Build history of the part. All positions in model axes, mm. Coordinates: 2 decimals unless noted, no trailing zeros. Loops run counter-clockwise (first coordinate to the right, second up) from the corner with the lowest first, then second, coordinate; pieces in that order, holes last.
Item 1: Cut at C-C (z = -2.5). List the corners of the cut face in (x, y), and give its area (3 significant figures).
Item 2: Cut at D-D (x = -1.5). List the corners of the cut face in (y, z), and give its area (3 significant figures).
Item 3: Flat gauge pin, fed straight in: pin 1 (2.5 mm diameter, centred on y = 0, z = 0, fed in from -X). Where does the tip first touch, or does it go through?
Item 4: Cut at A-A (y = -1). List the corners of the cut face in (x, z).
Item 5: Cut at B-B (z = 0.2). List the corners of the cut face in (x, y), and give its area (3 significant figures).
Item 6: Drill centre lines: line 1 along Z through (x, y) = (-1.1, -0.75); line 2 along Y through (x, z) = (1, 0); line 3 along Y through (x, z) = (-0.4, 0). Where is each one in solid material? Low to high.
from build123d import *
from build123d.topology import SkipClean

# Parameters (mm, degrees)
CUT_EXTRUDE_1_DEPTH      = 10
CUT_EXTRUDE_1_DEPTH_BACK = 10
SKETCH_2_W               = 8.130865192
SKETCH_2_H               = 8.836363256
SKETCH_2_W_2             = 5
SKETCH_2_H_2             = 6.113384394
SKETCH_3_R               = 1.5
CUT_EXTRUDE_2_DEPTH      = 10


with BuildPart() as part:
    # Sketch 1 → Revolve 1 (revolve)
    with SkipClean():  # the faces are left unmerged after this step: merging them gives an invalid solid
        with BuildSketch(Plane(origin=(0, 0, 0), x_dir=(1, 0, 0), z_dir=(0, 1, 0))):
            with BuildLine():
                ThreePointArc((3, 0), (2.121320344, 2.121320344), (0, 3))
                Line((0, 3), (0, -3))
                ThreePointArc((0, -3), (2.121320344, -2.121320344), (3, 0))
            make_face()
            with BuildLine():
                Line((0, -3), (0, 3))
                ThreePointArc((0, 3), (-3, 0), (0, -3))
            make_face()
        revolve(axis=Axis((0, 0, -3), (0, 0, 1)))

    # Sketch 2 → Cut-Extrude 1 (cut, two sides: drawn at the far end of the back side and taken through both)
    with SkipClean():  # the faces are left unmerged after this step: merging them gives an invalid solid
        with BuildSketch(Plane(origin=(0, 0, 0), x_dir=(1, 0, 0), z_dir=(0, 1, 0)).offset(-CUT_EXTRUDE_1_DEPTH_BACK)):
            with Locations((0.270511146, -0.599851934)):
                Rectangle(SKETCH_2_W, SKETCH_2_H)
            Rectangle(SKETCH_2_W_2, SKETCH_2_H_2, mode=Mode.SUBTRACT)
        extrude(amount=CUT_EXTRUDE_1_DEPTH + CUT_EXTRUDE_1_DEPTH_BACK, mode=Mode.SUBTRACT)

    # Sketch 3 → Cut-Extrude 2 (cut)
    with SkipClean():  # the faces are left unmerged after this step: merging them gives an invalid solid
        with BuildSketch(Plane(origin=(2.5, 0, 0), x_dir=(0, 0, -1), z_dir=(1, 0, 0))):
            Circle(SKETCH_3_R)
        extrude(amount=-CUT_EXTRUDE_2_DEPTH, mode=Mode.SUBTRACT)


solid = part.part
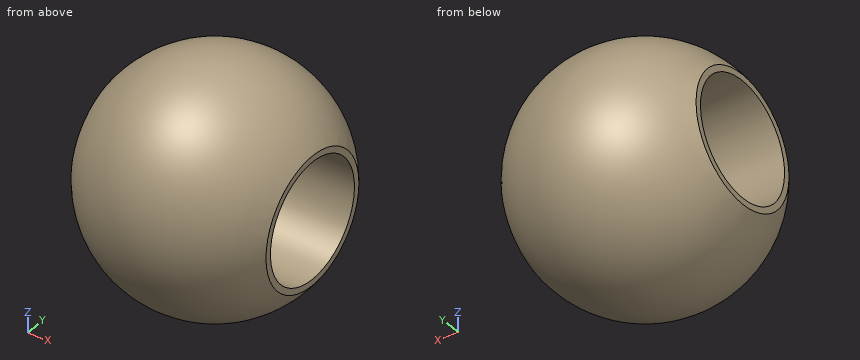
Filled sheet:
1. outline: circle Ø3.32 at (0, 0)
1. area: 8.64 mm2
2. outline: circle Ø5.2 at (0, 0); hole circle Ø3 at (0, 0)
2. area: 14.1 mm2
3. pin 1: passes through
4. outline: (-2.5, -1.32) arc R2.83 ccw to (2.5, -1.32) - (2.5, -1.12) - (-2.5, -1.12) - close; (-2.5, 1.12) - (2.5, 1.12) - (2.5, 1.32) arc R2.83 ccw to (-2.5, 1.32) - close
5. outline: (-2.5, -1.65) arc R2.99 ccw to (2.5, -1.65) - (2.5, -1.49) - (-2.5, -1.49) - close; (-2.5, 1.49) - (2.5, 1.49) - (2.5, 1.65) arc R2.99 ccw to (-2.5, 1.65) - close
5. area: 11.1 mm2
6. line 1: z = -2.69 to -1.3, 1.3 to 2.69
6. line 2: y = -2.83 to -1.5, 1.5 to 2.83
6. line 3: y = -2.97 to -1.5, 1.5 to 2.97
